```python
from build123d import *

# Parameters (mm, degrees)
SKETCH1_R      = 3.15
EXTRUDE1_DEPTH = 4


with BuildPart() as part:
    # Sketch1 → Extrude1 (new body)
    with BuildSketch(Plane.XY):
        Polygon((14.015385947, 97.315723434), (-15.984614053, 97.315723434), (-75.984614053, 37.315723434), (-75.984614053, 7.315723434), (14.015385947, 7.315723434), align=None)
        with Locations((-0.984614053, 52.315723434)):
            Circle(SKETCH1_R, mode=Mode.SUBTRACT)
        with Locations((-0.984614053, 82.315723434)):
            Circle(SKETCH1_R, mode=Mode.SUBTRACT)
        with Locations((-0.984614053, 22.315723434)):
            Circle(SKETCH1_R, mode=Mode.SUBTRACT)
        with Locations((-30.984614053, 22.315723434)):
            Circle(SKETCH1_R, mode=Mode.SUBTRACT)
        with Locations((-60.984614053, 22.315723434)):
            Circle(SKETCH1_R, mode=Mode.SUBTRACT)
    extrude(amount=EXTRUDE1_DEPTH)


solid = part.part
```
The listing builds one solid part. Answer for the finished solid, in the listing's coordinates (mm). Coordinates: 2 decimals unless noted, no trailing zeros. Write each loop counter-clockwise with the first axis right and the second up, starting at its lowest first coordinate (ties: lowest second). Pieces come first, ordered by that corner, then holes.
Q1. Section B-B, the plane y = 80.5 is taken. Write down the section's boundary in (x, z), then the cut area to 3 significant figures.
Returned:
outline: (-32.8, 0) - (-3.56, 0) - (-3.56, 4) - (-32.8, 4) - close; (1.59, 0) - (14.02, 0) - (14.02, 4) - (1.59, 4) - close
area: 167 mm2
Q2. Section A-A, the plane x = -29 is taken. Write down the section's boundary in (y, z), then the cut area to 3 significant figures.
Returned:
outline: (7.32, 0) - (19.87, 0) - (19.87, 4) - (7.32, 4) - close; (24.76, 0) - (84.3, 0) - (84.3, 4) - (24.76, 4) - close
area: 288 mm2
Q3. Section D-D, the plane z = 2.75 is taken. Write down the section's boundary in (x, y).
Returned:
outline: (-75.98, 7.32) - (14.02, 7.32) - (14.02, 97.32) - (-15.98, 97.32) - (-75.98, 37.32) - close; hole circle Ø6.3 at (-60.98, 22.32); hole circle Ø6.3 at (-30.98, 22.32); hole circle Ø6.3 at (-0.98, 22.32); hole circle Ø6.3 at (-0.98, 52.32); hole circle Ø6.3 at (-0.98, 82.32)
Q4. The mould has two halves that part along X. Classify faces 1 (the flat face through (14.015, 52, 2)), 2 (the flat face through (-1, 97.316, 2)), 3 (the cylindrical face through (-58.075, 21.109, 1.972)): released by +X, released by -X, zero draft, split by the parting line, or undercut.
Returned:
face 1: released by +X
face 2: zero draft
face 3: undercut
Q5. Given P1, Ø8, axis at x = -0.98, y = 52.32, coming from the +Z side; P2, Ø4, axis at x = -30.98, y = 22.32, coming from the -Z side; P3, Ø2, axis at y = 47, z = 1.5, coming from the -X side, each flat-ended and moving along its own axis, determine where each tip first touches the part or whether it passes through.
Returned:
P1: stops at z = 4
P2: passes through
P3: stops at x = -67.3
Q6. Section C-C, the plane x = -2 is taken. Write down the section's boundary in (y, z).
Returned:
outline: (7.32, 0) - (19.33, 0) - (19.33, 4) - (7.32, 4) - close; (25.3, 0) - (49.33, 0) - (49.33, 4) - (25.3, 4) - close; (55.3, 0) - (79.33, 0) - (79.33, 4) - (55.3, 4) - close; (85.3, 0) - (97.32, 0) - (97.32, 4) - (85.3, 4) - close
Q7. Find the intervals of material crossed by line 1 along Y through (x, z) = (0, 2.6); line 2 along X through (y, z) = (52.5, 1.2); line 3 along X through (y, z) = (53, 0.95), in increasing order.
Returned:
line 1: y = 7.32 to 19.32, 25.31 to 49.32, 55.31 to 79.32, 85.31 to 97.32
line 2: x = -60.8 to -4.13, 2.16 to 14.02
line 3: x = -60.3 to -4.06, 2.09 to 14.02
